```python
from build123d import *

# Parameters (mm, degrees)
SKETCH1_W           = 40.386
SKETCH1_H           = 19.558
BOSS_EXTRUDE1_DEPTH = 36.068
SKETCH2_W           = 7.627483077
SKETCH2_H           = 19.558
SKETCH2_R           = 1.5875
SKETCH2_W_2         = 7.627483076
BOSS_EXTRUDE2_DEPTH = 2.54
SKETCH3_R           = 4.064
BOSS_EXTRUDE3_DEPTH = 5.842


with BuildPart() as part:
    # Sketch1 → Boss-Extrude1 (new body)
    with BuildSketch(Plane.XY):
        with Locations((6770.286327778, 3542.568139787)):
            Rectangle(SKETCH1_W, SKETCH1_H)
    extrude(amount=BOSS_EXTRUDE1_DEPTH)

    # Sketch2 → Boss-Extrude2 (add)
    # profile 1 of 2: a face of its own
    with BuildSketch(Plane.XY.offset(28.956)):
        with Locations((6794.293069316, 3542.568139787)):
            Rectangle(SKETCH2_W, SKETCH2_H)
        with Locations((6794.416327778, 3537.488139787)):
            Circle(SKETCH2_R, mode=Mode.SUBTRACT)
        with Locations((6794.416327778, 3547.648139787)):
            Circle(SKETCH2_R, mode=Mode.SUBTRACT)
    # profile 2 of 2: a face of its own
    with BuildSketch(Plane.XY.offset(28.956)):
        with Locations((6746.27958624, 3542.568139787)):
            Rectangle(SKETCH2_W_2, SKETCH2_H)
        with Locations((6746.156327778, 3547.648139787)):
            Circle(SKETCH2_R, mode=Mode.SUBTRACT)
        with Locations((6746.156327778, 3537.488139787)):
            Circle(SKETCH2_R, mode=Mode.SUBTRACT)
    extrude(amount=-BOSS_EXTRUDE2_DEPTH)

    # Sketch3 → Boss-Extrude3 (add)
    with BuildSketch(Plane.XY.offset(36.068)):
        with Locations((6780.775840345, 3542.568139787)):
            Circle(SKETCH3_R)
    extrude(amount=BOSS_EXTRUDE3_DEPTH)


solid = part.part
```
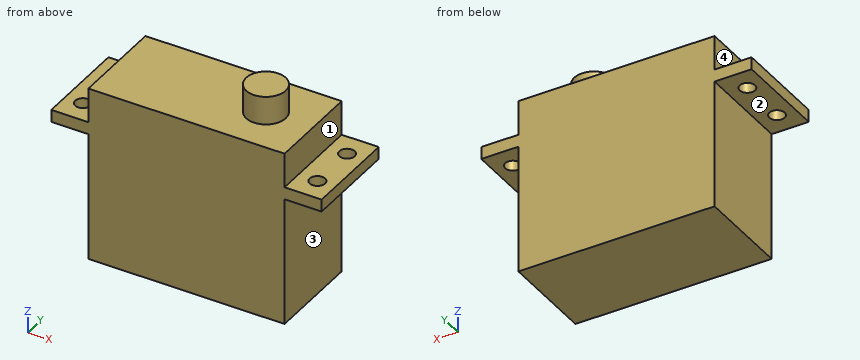
For this review, take the finished solid that the model builds, in its own axes (mm). Face numbers are marked on the shaded views. A direction names the side the tool comes from. Give positions to 0.01 mm unless a question says otherwise; leave off trailing zeros. Order: outer loops, then holes, each group sorted by start corner. A loop starts at its lowest first (then second) coordinate and runs counter-clockwise, first axis right, second up.
1) For the marked faces 1, 2, 3 and 4, list the 3-axis set-ups (+Z, -Z, +X, -X, +Y, -Y) from which the entire face can be reached by the end or side of a thin tool; tool diameter is ignored.
2) Take a section at B-B (x = 6781). Give the boundary of the cut face in (y, z).
3) Take a section at C-C (z = 21). Give the boundary of the cut face in (x, y).
4) Insertion check: pin 1 (1.5 mm diameter, centred on y = 3539, z = 12.5, fed in from +X); pin 2 (1 mm diameter, centred on y = 3542, z = 22, fed in from -X); pin 3 (2.5 mm diameter, centred on x = 6746.16, y = 3537.49, fed in from +Z); pin 4 (5 mm diameter, centred on x = 6794.42, y = 3547.65, fed in from +Z). Each pin has a flat end and moves straight along its axis. Give the tip position at first contact, or say it passes through.
5) Take a section at D-D (y = 3541.25). Give the boundary of the cut face in (x, z), then the cut area to 3 significant figures.
6) Take a section at A-A (y = 3535). Give the boundary of the cut face in (x, z).
7) Wall thickness on line 1 (X direction, y = 3547.5, z = 21); line 2 (Z direction, x = 6750, y = 3537); line 3 (Z direction, x = 6757, y = 3538.75): over which ranges is each line inside the solid? List them lowest first.
Derived:
1. face 1: +Z, +X, +Y, -Y
1. face 2: -Z, -X, +Y, -Y
1. face 3: -Z, +X, +Y, -Y
1. face 4: +Z, -X, +Y, -Y
2. outline: (3532.79, 0) - (3552.35, 0) - (3552.35, 36.07) - (3546.63, 36.07) - (3546.63, 41.91) - (3538.51, 41.91) - (3538.51, 36.07) - (3532.79, 36.07) - close
3. outline: (6750.09, 3532.79) - (6790.48, 3532.79) - (6790.48, 3552.35) - (6750.09, 3552.35) - close
4. pin 1: stops at x = 6790.48
4. pin 2: stops at x = 6750.09
4. pin 3: passes through
4. pin 4: stops at z = 28.96
5. outline: (6742.47, 26.42) - (6750.09, 26.42) - (6750.09, 0) - (6790.48, 0) - (6790.48, 26.42) - (6798.11, 26.42) - (6798.11, 28.96) - (6790.48, 28.96) - (6790.48, 36.07) - (6784.62, 36.07) - (6784.62, 41.91) - (6776.93, 41.91) - (6776.93, 36.07) - (6750.09, 36.07) - (6750.09, 28.96) - (6742.47, 28.96) - close
5. area: 1,540 mm2
6. outline: (6742.47, 26.42) - (6750.09, 26.42) - (6750.09, 0) - (6790.48, 0) - (6790.48, 26.42) - (6798.11, 26.42) - (6798.11, 28.96) - (6790.48, 28.96) - (6790.48, 36.07) - (6750.09, 36.07) - (6750.09, 28.96) - (6742.47, 28.96) - close
7. line 1: x = 6750.09 to 6790.48
7. line 2: z = 26.42 to 28.96
7. line 3: z = 0 to 36.07
